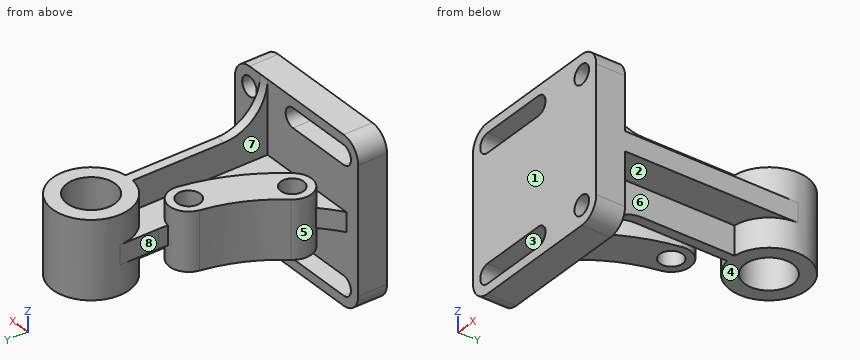
```python
from build123d import *

# Parameters (mm, degrees)
SKETCH1_W                            = 85
SKETCH1_H                            = 85
BOSS_EXTRUDE1_DEPTH                  = 15
SKETCH2_R                            = 20
BOSS_EXTRUDE2_DEPTH                  = 20
BOSS_EXTRUDE3_DEPTH                  = 5
BOSS_EXTRUDE4_DEPTH                  = 15
RIB1_START                           = -2.5
RIB1_DEPTH                           = 5
FILLET1_R                            = 10
F_10_0_10_DIAMETER_HOLE1_D           = 10
F_10_0_10_DIAMETER_HOLE1_CSINK_D     = 10.05
F_10_0_10_DIAMETER_HOLE1_CSINK_ANGLE = 90
CUT_EXTRUDE1_DEPTH                   = 126.349511367
CUT_EXTRUDE1_DEPTH_BACK              = 126.349511367
CUT_EXTRUDE2_DEPTH                   = 145.005208239
CUT_EXTRUDE2_DEPTH_BACK              = 145.005208239
SKETCH9_R                            = 12.5
SKETCH9_R_2                          = 6


with BuildPart() as part:
    # Sketch1 → Boss-Extrude1 (new body)
    with BuildSketch(Plane(origin=(0, 0, 0), x_dir=(1, 0, 0), z_dir=(0, 1, 0))):
        Rectangle(SKETCH1_W, SKETCH1_H)
    extrude(amount=BOSS_EXTRUDE1_DEPTH)



with BuildPart() as body_2:
    # Sketch2 → Boss-Extrude2 (new, symmetric)
    with BuildSketch(Plane.XY):
        with Locations((22.5, 105)):
            Circle(SKETCH2_R)
    extrude(amount=BOSS_EXTRUDE2_DEPTH, both=True)


with BuildPart() as part_1:
    add(part.part)

    add(body_2.part)  # Boss-Extrude3 merges body 2
    # Sketch4 → Boss-Extrude3 (add, symmetric)
    with BuildSketch(Plane.XY):
        with BuildLine():
            Line((42.5, 105), (42.5, 15))
            Line((42.5, 15), (-34.281746195, 15))
            ThreePointArc((-34.281746195, 15), (-7.255227512, 45.462369655), (2.5, 85))
            Line((2.5, 85), (2.5, 105))
            ThreePointArc((2.5, 105), (22.5, 85), (42.5, 105))
        make_face()
    extrude(amount=BOSS_EXTRUDE3_DEPTH, both=True)

    # Sketch5 → Boss-Extrude4 (add, symmetric)
    with BuildSketch(Plane.XY):
        with BuildLine():
            ThreePointArc((-9.725777904, 23.93517708), (3.599239768, 44.851265135), (11.056736536, 68.503423122))
            ThreePointArc((11.056736536, 68.503423122), (2.945140783, 80.087982428), (-8.639418524, 71.976386675))
            ThreePointArc((-8.639418524, 71.976386675), (-14.526915972, 53.303630369), (-25.046666766, 36.790929274))
            ThreePointArc((-25.046666766, 36.790929274), (-23.814098432, 22.702608745), (-9.725777904, 23.93517708))
        make_face()
    extrude(amount=BOSS_EXTRUDE4_DEPTH, both=True)

    # Rib1: read off the stored shape, not the designer's step
    # Rib1 outline → Rib1 (add)
    with BuildSketch(Plane(origin=(22.5, 0, 0), x_dir=(0, 0, -1), z_dir=(1, 0, 0)).offset(RIB1_START)):
        with BuildLine():
            Line((-5, 15), (-5, 85.156865167))
            Line((-5, 85.156865167), (-20, 85.156865167))
            Line((-20, 85.156865167), (-20, 37.5))
            ThreePointArc((-20, 37.5), (-26.590097423, 21.590097423), (-42.5, 15))
            Line((-42.5, 15), (-5, 15))
        make_face()
    rib1 = extrude(amount=RIB1_DEPTH)

    # Mirror1: Rib1 across plane
    add(rib1.mirror(Plane.XY))

    # Fillet1
    fillet1_edges = [part_1.edges().sort_by_distance(p)[0] for p in [
        (42.5, 7.5, 42.5),
        (-42.5, 7.5, 42.5),
        (-42.5, 7.5, -42.5),
        (42.5, 7.5, -42.5),
    ]]
    fillet(fillet1_edges, radius=FILLET1_R)

    # Ø10.0 (10) Diameter Hole1 (through all)
    with Locations(Plane(origin=(32.5, 15, -32.5), x_dir=(0, 0, 1), z_dir=(0, 1, 0))):
        with Locations((0, 0), (65, 0)):
            CounterSinkHole(F_10_0_10_DIAMETER_HOLE1_D / 2, F_10_0_10_DIAMETER_HOLE1_CSINK_D / 2, counter_sink_angle=F_10_0_10_DIAMETER_HOLE1_CSINK_ANGLE)

    # Sketch8 → Cut-Extrude1 (cut, two sides: drawn at the far end of the back side and taken through both)
    with BuildSketch(Plane(origin=(0, 15, 0), x_dir=(1, 0, 0), z_dir=(0, 1, 0)).offset(-CUT_EXTRUDE1_DEPTH_BACK)):
        with BuildLine():
            Line((-32.5, -27.5), (2.5, -27.5))
            ThreePointArc((2.5, -27.5), (7.5, -32.5), (2.5, -37.5))
            Line((2.5, -37.5), (-32.5, -37.5))
            ThreePointArc((-32.5, -37.5), (-37.5, -32.5), (-32.5, -27.5))
        make_face()
        with BuildLine():
            Line((-32.5, 27.5), (2.5, 27.5))
            ThreePointArc((2.5, 27.5), (7.5, 32.5), (2.5, 37.5))
            Line((2.5, 37.5), (-32.5, 37.5))
            ThreePointArc((-32.5, 37.5), (-37.5, 32.5), (-32.5, 27.5))
        make_face()
    extrude(amount=CUT_EXTRUDE1_DEPTH + CUT_EXTRUDE1_DEPTH_BACK, mode=Mode.SUBTRACT)

    # Sketch9 → Cut-Extrude2 (cut, two sides: drawn at the far end of the back side and taken through both)
    with BuildSketch(Plane.XY.offset(15).offset(-CUT_EXTRUDE2_DEPTH_BACK)):
        with Locations((22.5, 105)):
            Circle(SKETCH9_R)
        with Locations((1.208659006, 70.239904898)):
            Circle(SKETCH9_R_2)
        with Locations((-17.386222335, 30.363053177)):
            Circle(SKETCH9_R_2)
    extrude(amount=CUT_EXTRUDE2_DEPTH + CUT_EXTRUDE2_DEPTH_BACK, mode=Mode.SUBTRACT)


solid = part_1.part
```
Design review of the part built by this model. Coordinates are the model's own, in mm. Face numbers are marked on the shaded views. A direction names the side the tool comes from. Give positions to 0.01 mm unless a question says otherwise; leave off trailing zeros. Loops run counter-clockwise (first coordinate to the right, second up) from the corner with the lowest first, then second, coordinate; pieces in that order, holes last. Notation, with made-up numbers: (22, 55.25) -> (51, 55.25) arc R22 ccw to (51, 84.25) -> close; hole circle Ø6 at (73.25, 71.25). An arc over 180 degrees is marked (long way). Write each question's results on one line, items separated by ' | '.
Q1. The part is to be moulded in two halves that separate along Z. For the marked faces 1, 2 and 3, say which applies: +Z half, -Z half, draft (parallel to the pull), parting line (faces both ways), or undercut.
Reply:
face 1: draft | face 2: -Z half | face 3: undercut
Q2. Take a section at D-D, the plane y = 97. Write out the cut boundary in (x, z), plus the area to 3 significant figures.
Reply:
outline: (2.5, -5) -> (4.17, -5) -> (4.17, -20) -> (12.9, -20) -> (12.9, 20) -> (4.17, 20) -> (4.17, 5) -> (2.5, 5) -> close; (32.1, -20) -> (40.83, -20) -> (40.83, -5) -> (42.5, -5) -> (42.5, 5) -> (40.83, 5) -> (40.83, 20) -> (32.1, 20) -> close | area: 731 mm²
Q3. Wall thickness on L1, parallel to Z at x = 32.5, y = 3.75; L2, parallel to X at y = 11.25, z = 32.5; L3, parallel to Y at x = 13, z = 24: over which ranges is each line inside the solid? List them lowest first.
Reply:
L1: z = -42.5 to -37.5, -27.5 to 27.5, 37.5 to 42.5 | L2: x = -42.5 to -37.5, 7.5 to 27.5, 37.5 to 42.5 | L3: y = 0 to 15
Q4. Take a section at B-B, the plane y = 10.5. Write out the cut boundary in (x, z).
Reply:
outline: (-42.5, -32.5) arc R10 ccw to (-32.5, -42.5) -> (32.5, -42.5) arc R10 ccw to (42.5, -32.5) -> (42.5, 32.5) arc R10 ccw to (32.5, 42.5) -> (-32.5, 42.5) arc R10 ccw to (-42.5, 32.5) -> close; hole (-32.5, -37.5) -> (2.5, -37.5) arc R5 ccw to (2.5, -27.5) -> (-32.5, -27.5) arc R5 ccw to start; hole (-32.5, 27.5) -> (2.5, 27.5) arc R5 ccw to (2.5, 37.5) -> (-32.5, 37.5) arc R5 ccw to start; hole circle Ø10 at (32.5, -32.5); hole circle Ø10 at (32.5, 32.5)
Q5. Take a section at A-A, the plane x = 22.5. Write out the cut boundary in (y, z).
Reply:
outline: (0, -42.5) -> (15, -42.5) arc R22.5 cw to (37.5, -20) -> (92.5, -20) -> (92.5, 20) -> (37.5, 20) arc R22.5 cw to (15, 42.5) -> (0, 42.5) -> close; (117.5, -20) -> (125, -20) -> (125, 20) -> (117.5, 20) -> close
Q6. Machinability: for the marked faces 4, 5, 6, 7 and 8, which of the approach directions +Z, -Z, +X, -X, +Y, -Y give a long, thin tool a straight path to every point of the face, cutting with its end or side? Answer none if there is none.
Reply:
face 4: -Z, +X, -X, +Y | face 5: none | face 6: -Z, +X | face 7: +Z | face 8: +Z, -Z, -X, +Y
Q7. Take a section at C-C, the plane y = 83. Write out the cut boundary in (x, z).
Reply:
outline: (2.48, -5) -> (20, -5) -> (20, -20) -> (25, -20) -> (25, -5) -> (42.5, -5) -> (42.5, 5) -> (25, 5) -> (25, 20) -> (20, 20) -> (20, 5) -> (2.48, 5) -> close
Q8. For pin 1 Ø11 at (y, z) = (34, 21.5) entering from -X; pin 2 Ø14 at (x, z) = (30.5, -30) entering from +Y; pin 3 Ø19 at (x, y) = (-17.39, 30.36) entering from -Z; pin 4 Ø9 at (x, z) = (32.5, -32.5) entering from -Y, all flat-tipped, find the tip position at first contact; note any pin that passes through.
Reply:
pin 1: stops at x = 20 | pin 2: stops at y = 22.57 | pin 3: stops at z = -15 | pin 4: passes through
